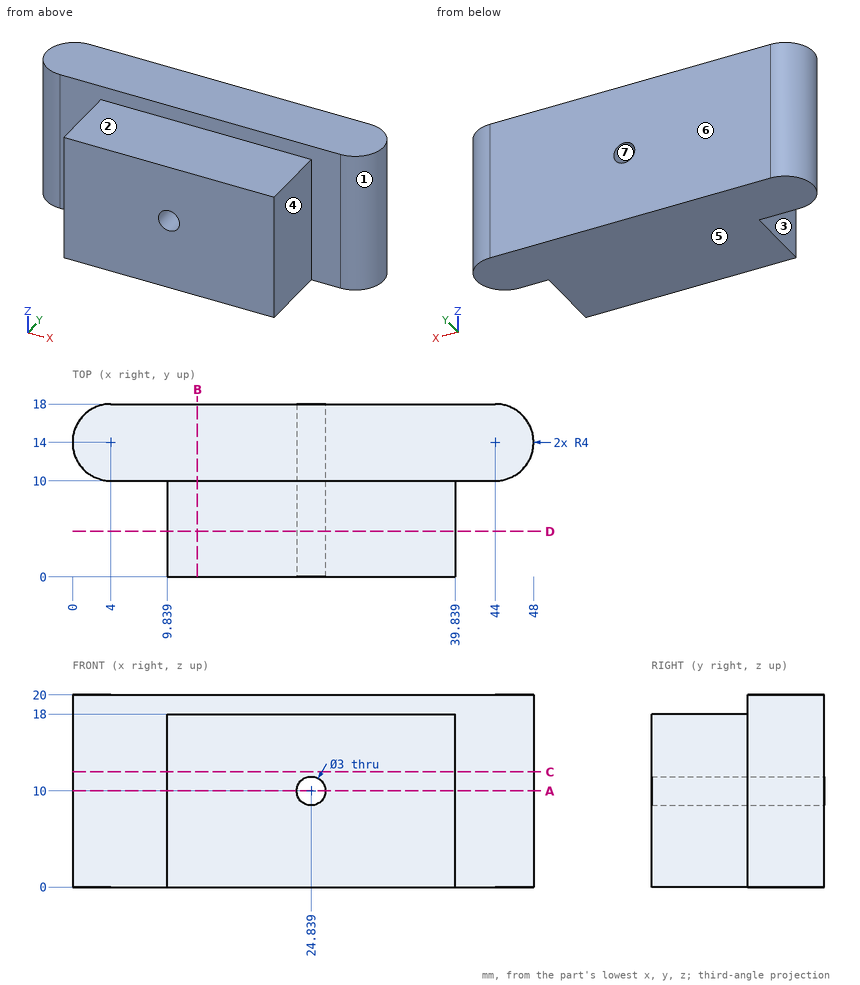
Answer from the drawing. Dimensions are ordinates in mm from the lowest x, y and z of the part. A direction names the side the tool comes from. Round coordinates to 2 decimals unless told otherwise and drop trailing zeros. Write each loop counter-clockwise with the first axis right and the second up, starting at its lowest first coordinate (ties: lowest second). Pieces come first, ordered by that corner, then holes. Notation, with made-up numbers: (-1.5, 16.5) -> (28.5, 16.5) arc R12 ccw to (28.5, 20.5) -> close; hole circle Ø1 at (40, 7). An arc over 180 degrees is marked (long way). Answer in a Markdown table with one row per item. Add a question column.
1) Determine the mould class of the marked faces 5, 6 and 7 for opening direction Z: pulls with the +Z half, pulls with the -Z half, needs draft (parallel to the pull), parting line crosses it, or undercut.
2) Find section B-B, the plane x = 13. Determine the outline of the cut face in (y, z).
3) Find section D-D, the plane y = 4.75. Determine the outline of the cut face in (x, z), and give its area (3 significant figures).
4) Find section A-A, the plane z = 10. Determine the outline of the cut face in (x, y).
5) Find section C-C, the plane z = 12. Determine the outline of the cut face in (x, y), and give its area (3 significant figures).
6) Consider line 1 (Z direction, x = 25, y = 15); line 2 (X direction, y = 2, z = 7.5); line 3 (Y direction, x = 15, z = 19.25). Determine where each line is inside the solid, lowest interval first.
7) Given P1, Ø10, axis at y = 4, z = 12, coming from the -X side; P2, Ø5, axis at y = 2.5, z = 3.5, coming from the +X side; P3, Ø3, axis at x = 7, z = 6, coming from the -Y side, each flat-ended and moving along its own axis, determine where each tip first touches the part or whether it passes through.
8) Which of the six approach directions +Z, -Z, +X, -X, +Y, -Y give full straight-line access (tool end or side, diameter ignored) to the marked faces 1, 2, 3 and 4?
Findings below:
| question | item | result |
|---|---|---|
| 1 | face 5 | pulls with the -Z half |
| 1 | face 6 | needs draft |
| 1 | face 7 | undercut |
| 2 | outline | (0, 0) -> (18, 0) -> (18, 20) -> (10, 20) -> (10, 18) -> (0, 18) -> close |
| 3 | outline | (9.84, 0) -> (39.84, 0) -> (39.84, 18) -> (9.84, 18) -> close; hole circle Ø3 at (24.84, 10) |
| 3 | area | 533 mm² |
| 4 | outline | (4, 10) -> (9.84, 10) -> (9.84, 0) -> (23.34, 0) -> (23.34, 18) -> (4, 18) arc R4 ccw to start; (26.34, 0) -> (39.84, 0) -> (39.84, 10) -> (44, 10) arc R4 ccw to (44, 18) -> (26.34, 18) -> close |
| 5 | outline | (4, 10) -> (9.84, 10) -> (9.84, 0) -> (39.84, 0) -> (39.84, 10) -> (44, 10) arc R4 ccw to (44, 18) -> (4, 18) arc R4 ccw to start |
| 5 | area | 670 mm² |
| 6 | line 1 | 0 to 8.51, 11.49 to 20 |
| 6 | line 2 | 9.84 to 39.84 |
| 6 | line 3 | 10 to 18 |
| 7 | P1 | x = 9.84 |
| 7 | P2 | x = 39.84 |
| 7 | P3 | y = 10 |
| 8 | face 1 | +Z, -Z, +X |
| 8 | face 2 | +Z, +X, -X, -Y |
| 8 | face 3 | +Z, -Z, -X, -Y |
| 8 | face 4 | +Z, -Z, +X, -Y |
